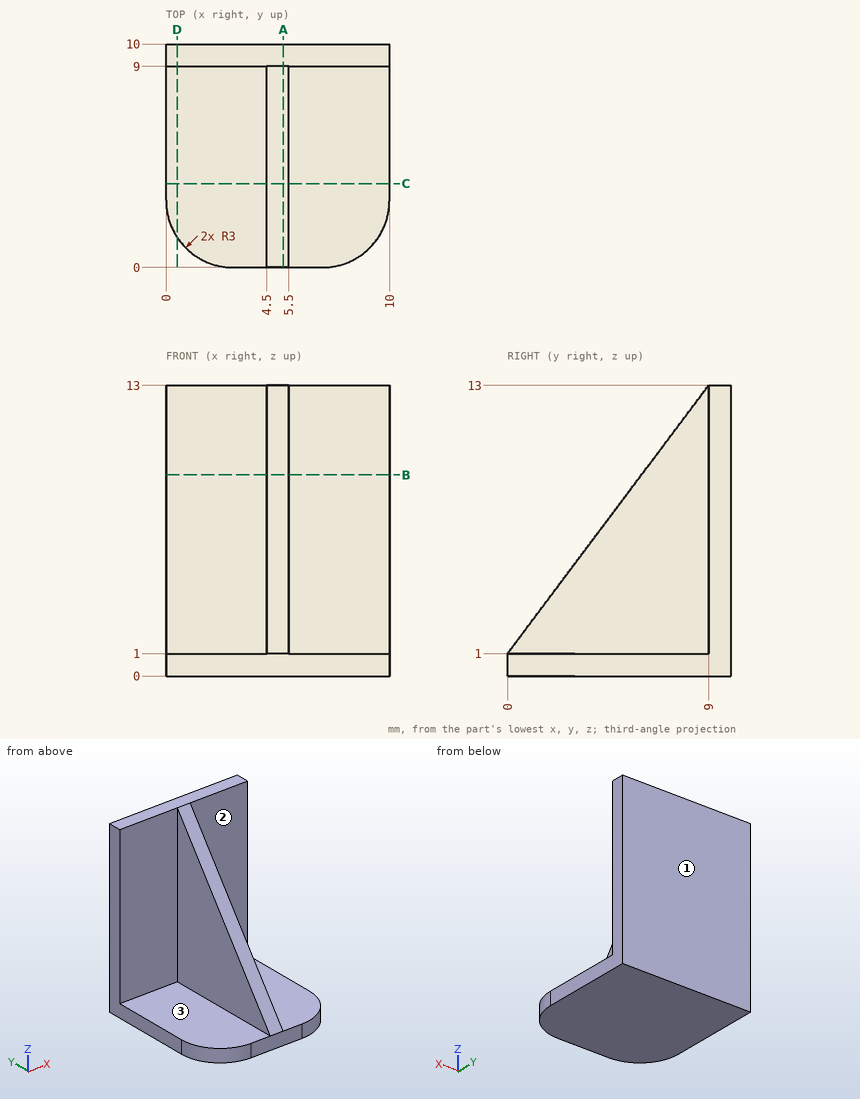
Can you work these out from the drawing? Everything is in mm from the part's minimum corner. A direction names the side the tool comes from. Give positions to 0.01 mm unless a question says otherwise; leave off trailing zeros. Order: outer loops, then holes, each group sorted by start corner. A loop starts at its lowest first (then second) coordinate and runs counter-clockwise, first axis right, second up.
Item 1: I'm going to push flat-ended pins straight in: pin 1 (2 mm diameter, centred on y = 1, z = 5.5, fed in from +X); pin 2 (2 mm diameter, centred on x = 2.5, z = 6, fed in from -Y); pin 3 (3 mm diameter, centred on x = 4, y = 8.5, fed in from +Z); pin 4 (5 mm diameter, centred on x = 2.5, y = 1.5, fed in from +Z). Where does each tip first touch, or does it pass through?
Item 2: If we section it at B-B, the plane z = 9: Write out the boundary of the cut face in (x, y).
Item 3: For the marked faces 1, 2 and 3, which set-ups out of +Z, -Z, +X, -X, +Y, -Y let a thin tool reach every point of the face, with its end or its side?
Item 4: If we section it at A-A, the plane x = 5.25: Write out the boundary of the cut face in (y, z), plus the area to 3 significant figures.
Item 5: If we section it at D-D, the plane x = 0.5: Write out the boundary of the cut face in (y, z), plus the area to 3 significant figures.
Item 6: If we section it at C-C, the plane y = 3.75: Write out the boundary of the cut face in (x, z).
Item 7: I need wall thicknesses on line 1 (X direction, y = 2.25, z = 1.5); line 2 (Z direction, x = 1, y = 5); line 3 (Y direction, x = 9, z = 7). Which ranges of each line are inside material? Lowest first, please.
Values:
1. pin 1: passes through
1. pin 2: stops at y = 9
1. pin 3: stops at z = 13
1. pin 4: stops at z = 5
2. outline: (0, 9) - (4.5, 9) - (4.5, 6) - (5.5, 6) - (5.5, 9) - (10, 9) - (10, 10) - (0, 10) - close
3. face 1: +Z, -Z, +X, -X, +Y
3. face 2: +Z, +X, -Y
3. face 3: +Z, -X, -Y
4. outline: (0, 0) - (10, 0) - (10, 13) - (9, 13) - (0, 1) - close
4. area: 76.0 mm2
5. outline: (1.34, 0) - (10, 0) - (10, 13) - (9, 13) - (9, 1) - (1.34, 1) - close
5. area: 20.7 mm2
6. outline: (0, 0) - (10, 0) - (10, 1) - (5.5, 1) - (5.5, 6) - (4.5, 6) - (4.5, 1) - (0, 1) - close
7. line 1: x = 4.5 to 5.5
7. line 2: z = 0 to 1
7. line 3: y = 9 to 10
